Check sheet for the modelled part. Datum: model origin and axes. Units: mm. Face numbers are marked on the shaded views. A direction names the side the tool comes from. Give positions to 0.01 mm unless a question says otherwise; leave off trailing zeros. Order: outer loops, then holes, each group sorted by start corner. A loop starts at its lowest first (then second) coordinate and runs counter-clockwise, first axis right, second up. Notation, with made-up numbers: (17, 36.5) -> (62, 36.5) arc R9 ccw to (62, 46.5) -> close; hole circle Ø11 at (34, 42). An arc over 180 degrees is marked (long way). Write each question's results on one line, items separated by ' | '.
from build123d import *
from build123d.topology import SkipClean

# Parameters (mm, degrees)
BOSS_EXTRUDE1_DEPTH = 2.5
BOSS_EXTRUDE2_START = -2.5
SKETCH1_3_W         = 15
SKETCH1_3_H         = 40
SKETCH1_3_R         = 1.7
SKETCH1_3_R_2       = 1.6
BOSS_EXTRUDE2_DEPTH = 2.5
CUT_EXTRUDE1_DEPTH  = 2.5
BOSS_EXTRUDE3_START = 1
SKETCH2_R           = 1.6
BOSS_EXTRUDE3_DEPTH = 1


with BuildPart() as part:
    # Sketch1 → Boss-Extrude1 (new body)
    with BuildSketch(Plane(origin=(0, 0, 0), x_dir=(0, 0, -1), z_dir=(1, 0, 0))):
        with BuildLine():
            Line((7.5, 21.7), (7.5, 40))
            Line((7.5, 40), (0, 40))
            Line((0, 40), (0, 0))
            Line((0, 0), (7.5, 0))
            Line((7.5, 0), (7.5, 6.4))
            ThreePointArc((7.5, 6.4), (5.9, 8), (7.5, 9.6))
            Line((7.5, 9.6), (7.5, 18.3))
            ThreePointArc((7.5, 18.3), (5.8, 20), (7.5, 21.7))
        make_face()
        with BuildLine():
            Line((15, 40), (7.5, 40))
            Line((7.5, 40), (7.5, 21.7))
            ThreePointArc((7.5, 21.7), (8.702081528, 21.202081528), (9.2, 20))
            ThreePointArc((9.2, 20), (8.702081528, 18.797918472), (7.5, 18.3))
            Line((7.5, 18.3), (7.5, 9.6))
            ThreePointArc((7.5, 9.6), (8.63137085, 9.13137085), (9.1, 8))
            ThreePointArc((9.1, 8), (8.63137085, 6.86862915), (7.5, 6.4))
            Line((7.5, 6.4), (7.5, 0))
            Line((7.5, 0), (15, 0))
            Line((15, 0), (15, 5.883419246))
            Line((15, 5.883419246), (12.2, 4.266838493))
            Line((12.2, 4.266838493), (9.4, 5.883419246))
            Line((9.4, 5.883419246), (9.4, 9.116580754))
            Line((9.4, 9.116580754), (12.2, 10.733161507))
            Line((12.2, 10.733161507), (15, 9.116580754))
            Line((15, 9.116580754), (15, 30.883419246))
            Line((15, 30.883419246), (12.2, 29.266838493))
            Line((12.2, 29.266838493), (9.4, 30.883419246))
            Line((9.4, 30.883419246), (9.4, 34.116580754))
            Line((9.4, 34.116580754), (12.2, 35.733161507))
            Line((12.2, 35.733161507), (15, 34.116580754))
            Line((15, 34.116580754), (15, 40))
        make_face()
        with BuildLine():
            ThreePointArc((9.1, 8), (8.63137085, 9.13137085), (7.5, 9.6))
            Line((7.5, 9.6), (7.5, 6.4))
            ThreePointArc((7.5, 6.4), (8.63137085, 6.86862915), (9.1, 8))
        make_face()
        with BuildLine():
            Line((7.5, 6.4), (7.5, 9.6))
            ThreePointArc((7.5, 9.6), (5.9, 8), (7.5, 6.4))
        make_face()
    extrude(amount=BOSS_EXTRUDE1_DEPTH)

    # Sketch1_3 → Boss-Extrude2 (add)
    with SkipClean():  # the faces are left unmerged after this step: merging them gives an invalid solid
        with BuildSketch(Plane(origin=(0, 0, 0), x_dir=(0, 0, -1), z_dir=(1, 0, 0)).offset(BOSS_EXTRUDE2_START)):
            with Locations((7.5, 20)):
                Rectangle(SKETCH1_3_W, SKETCH1_3_H)
            with Locations((7.5, 20)):
                Circle(SKETCH1_3_R, mode=Mode.SUBTRACT)
            with Locations((12.2, 32.5)):
                Circle(SKETCH1_3_R_2, mode=Mode.SUBTRACT)
            with Locations((12.2, 7.5)):
                Circle(SKETCH1_3_R_2, mode=Mode.SUBTRACT)
        extrude(amount=BOSS_EXTRUDE2_DEPTH)

    # Sketch3 → Cut-Extrude1 (cut)
    with SkipClean():  # the faces are left unmerged after this step: merging them gives an invalid solid
        with BuildSketch(Plane.ZY.offset(2.5)):
            with BuildLine():
                ThreePointArc((0, 33.564659966), (-2.979157617, 27.071067812), (-4, 20))
                Line((-4, 20), (0, 20))
                Line((0, 20), (0, 33.564659966))
            make_face()
            with BuildLine():
                Line((0, 20), (-4, 20))
                ThreePointArc((-4, 20), (-2.979157617, 12.928932188), (0, 6.435340034))
                Line((0, 6.435340034), (0, 20))
            make_face()
            with BuildLine():
                Line((0, 33.564659966), (0, 20))
                Line((0, 20), (0, 6.435340034))
                ThreePointArc((0, 6.435340034), (28.071067812, -3.979157617), (46, 20))
                ThreePointArc((46, 20), (28.071067812, 43.979157617), (0, 33.564659966))
            make_face()
        extrude(amount=-CUT_EXTRUDE1_DEPTH, mode=Mode.SUBTRACT)

    # Sketch2 → Boss-Extrude3 (add)
    # profile 1 of 2: a face of its own
    with SkipClean():  # the faces are left unmerged after this step: merging them gives an invalid solid
        with BuildSketch(Plane.ZY.offset(2.5).offset(BOSS_EXTRUDE3_START)):
            with BuildLine():
                ThreePointArc((-8.6, 32.5), (-11, 35.89411255), (-15, 34.7627417))
                Line((-15, 34.7627417), (-15, 30.2372583))
                ThreePointArc((-15, 30.2372583), (-11, 29.10588745), (-8.6, 32.5))
            make_face()
            with Locations(Location((-12.2, 32.5, 0), (0, 0, 180))):
                Circle(SKETCH2_R, mode=Mode.SUBTRACT)
        # profile 2 of 2: a face of its own
        with BuildSketch(Plane.ZY.offset(2.5).offset(BOSS_EXTRUDE3_START)):
            with BuildLine():
                ThreePointArc((-8.6, 7.5), (-11, 10.89411255), (-15, 9.7627417))
                Line((-15, 9.7627417), (-15, 5.2372583))
                ThreePointArc((-15, 5.2372583), (-11, 4.10588745), (-8.6, 7.5))
            make_face()
            with Locations(Location((-12.2, 7.5, 0), (0, 0, 180))):
                Circle(SKETCH2_R, mode=Mode.SUBTRACT)
        extrude(amount=-BOSS_EXTRUDE3_DEPTH)


solid = part.part
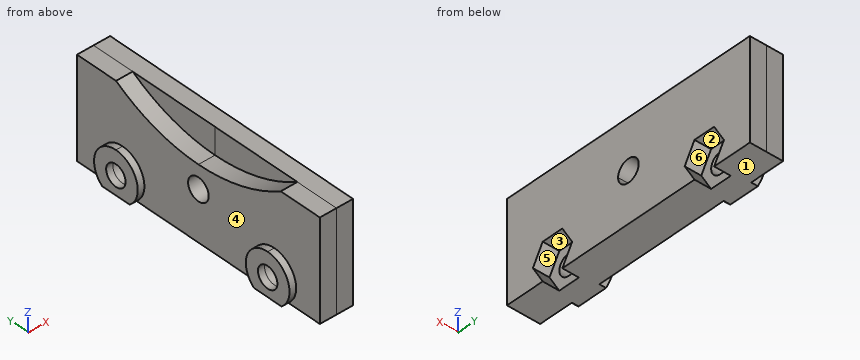
1. Material ranges on probe 1 along Y at (x, z) = (-2.9, -12.2); probe 2 along Y at (x, z) = (-1.1, -12.2); probe 3 along Y at (x, z) = (-0.65, -13.5), recorded low to high. Write a range as from..to.
Verdict:
probe 1: y = 3.9..5.9, 9.1..11.1, 28.9..30.9, 34.1..36.1 | probe 2: y = 0..5.9, 9.1..30.9, 34.1..40 | probe 3: y = 0..6.57, 8.43..31.57, 33.43..40
2. Section check D-D on y = 15.5. Record the cut outline in (x, z), then the cut area to 3 significant figures.
Verdict:
outline: (-2.5, -15) -> (2.5, -15) -> (2.5, 0) -> (0, 0) -> (0, -3.59) -> (-2.5, -3.59) -> close | area: 66.0 mm^2
3. Mould release check, pull along Z, two halves, no side actions. Record for the marked faces 3, 4, 5 and 6: +Z half, -Z half, draft (parallel to the pull), parting line (faces both ways), or undercut.
Verdict:
face 3: -Z half | face 4: draft | face 5: undercut | face 6: undercut
4. Section check B-B on z = -3. Record the cut outline in (x, y).
Verdict:
outline: (-2.5, 0) -> (2.5, 0) -> (2.5, 40) -> (-2.5, 40) -> (-2.5, 27) -> (0, 27) -> (0, 13) -> (-2.5, 13) -> close
5. Section check A-A on x = -0.9. Record the cut outline in (y, z), then the cut area to 3 significant figures.
Verdict:
outline: (0, -15) -> (40, -15) -> (40, 0) -> (33.56, 0) arc R25 cw to (6.44, 0) -> (0, 0) -> close; hole circle Ø3.2 at (7.5, -12.2); hole circle Ø3.4 at (20, -7.5); hole circle Ø3.2 at (32.5, -12.2) | area: 501 mm^2
6. Access from +Z, -Z, +X, -X, +Y, -Y to the whole of each face (thin tool, end or side, straight path). Record for the marked faces 1 and 2.
Verdict:
face 1: -Z, +X, -X, +Y, -Y | face 2: -Z, +X
7. Section check C-C on y = 7. Record the cut outline in (x, z).
Verdict:
outline: (-3.5, -15) -> (0, -15) -> (0, -13.72) -> (-3.5, -13.72) -> close; (-3.5, -10.68) -> (0, -10.68) -> (0, -9.4) -> (2.5, -9.4) -> (2.5, 0) -> (0, 0) -> (0, -0.35) -> (-2.5, -0.35) -> (-2.5, -8.63) -> (-3.5, -8.63) -> close
8. Gauge pin test, flat ends, axial feed: pin 1 Ø6 at (y, z) = (23.5, -13) entering from -X; pin 2 Ø2 at (y, z) = (25.5, -1.5) entering from -X. Record the tip position at first contact, or that the pin passes through.
Verdict:
pin 1: stops at x = -2.5 | pin 2: stops at x = 0
